Input: dimensioned drawing with shaded views. Units: mm. Origin: part minimum x, y, z. A direction names the side the tool comes from. Give positions to 0.01 mm unless a question says otherwise; leave off trailing zeros. Order: outer loops, then holes, each group sorted by start corner. A loop starts at its lowest first (then second) coordinate and runs counter-clockwise, first axis right, second up.
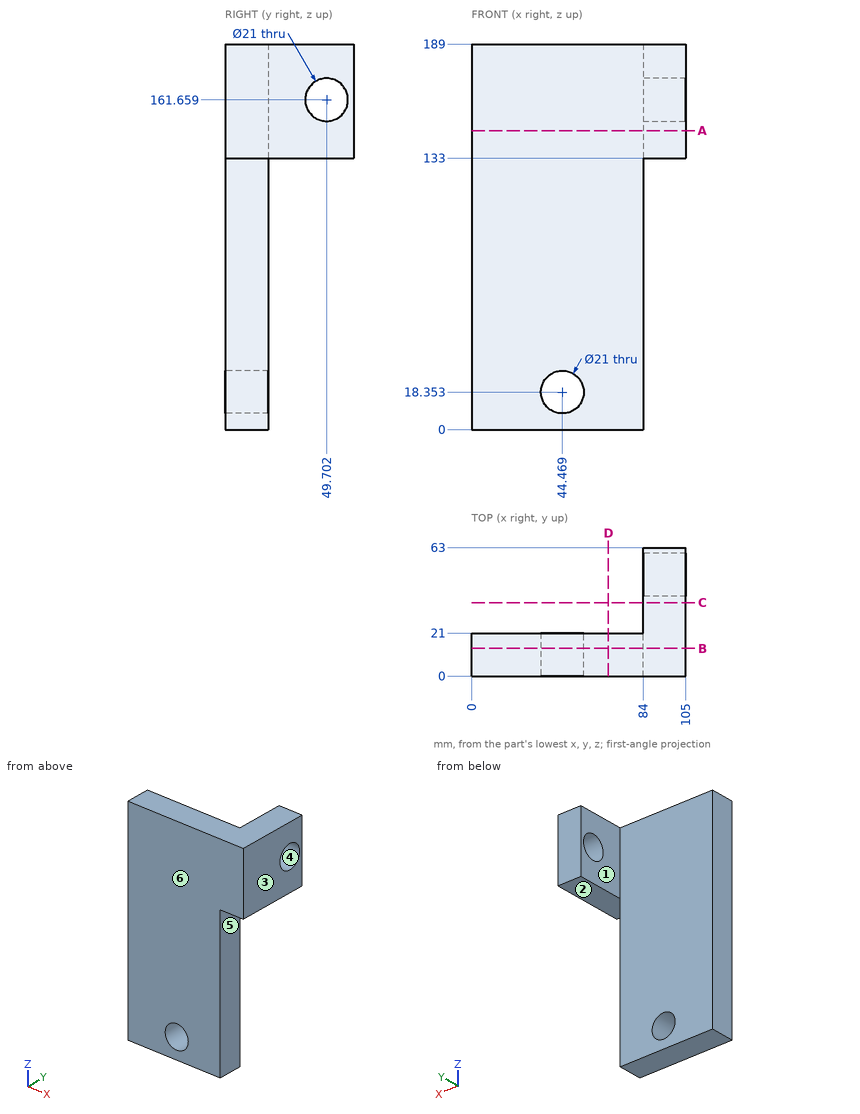
1) Draft query along Y for the marked faces 4, 5 and 6. Return one class per face: +Y half, -Y half, draft (parallel to the pull), parting line (faces both ways), or undercut.
Report:
face 4: undercut
face 5: draft
face 6: -Y half
2) Reachability of the marked faces 1, 2 and 3 from +Z, -Z, +X, -X, +Y, -Y: full face, straight path, thin tool, end or side. Return the list, or none.
Report:
face 1: +Z, -Z, -X, +Y
face 2: -Z, +X, +Y, -Y
face 3: +Z, -Z, +X, +Y, -Y
3) Section query C-C, the plane y = 36. Return the cut outline in (x, z), and give its area (3 significant figures).
Report:
outline: (84, 133) - (105, 133) - (105, 189) - (84, 189) - close
area: 1,180 mm2
4) Section query A-A, the plane z = 146.5. Return the cut outline in (x, y).
Report:
outline: (0, 0) - (105, 0) - (105, 63) - (84, 63) - (84, 21) - (0, 21) - close
5) Section query D-D, the plane x = 67. Return the cut outline in (y, z), and give its area (3 significant figures).
Report:
outline: (0, 0) - (21, 0) - (21, 189) - (0, 189) - close
area: 3,970 mm2
6) Section query B-B, the plane y = 13.5. Return the cut outline in (x, z), and give its area (3 significant figures).
Report:
outline: (0, 0) - (84, 0) - (84, 133) - (105, 133) - (105, 189) - (0, 189) - close; hole circle Ø21 at (44.47, 18.35)
area: 16,700 mm2
7) Material intervals for L1, parallel to Y at x = 41.5, z = 108.5; L2, parallel to Z at x = 97.5, y = 13; L3, parallel to Z at x = 43.5, y = 8.5, sorted ascending.
Report:
L1: y = 0 to 21
L2: z = 133 to 189
L3: z = 0 to 7.9, 28.81 to 189
8) Pin query (flat end, axial travel): pin 1 (23 mm diameter, centred on x = 96, y = 31.5, fed in from -Z); pin 2 (12.5 mm diameter, centred on y = 44.5, z = 171.5, fed in from -X); pin 3 (17 mm diameter, centred on y = 8, z = 47.5, fed in from +X). Return the tip coordinate at first contact, or that it passes through.
Report:
pin 1: stops at z = 133
pin 2: stops at x = 84
pin 3: stops at x = 84
